The listing builds one solid part. Answer for the finished solid, in the listing's coordinates (mm). Face numbers are marked on the shaded views. Coordinates: 2 decimals unless noted, no trailing zeros. Write each loop counter-clockwise with the first axis right and the second up, starting at its lowest first coordinate (ties: lowest second). Pieces come first, ordered by that corner, then holes. Notation, with made-up numbers: M -10,-25 L 23,-25 A19 cw 23,-21 Z; hole C 87,36.25 d2. An arc over 180 degrees is marked long. Answer as CSV lines item,"result".
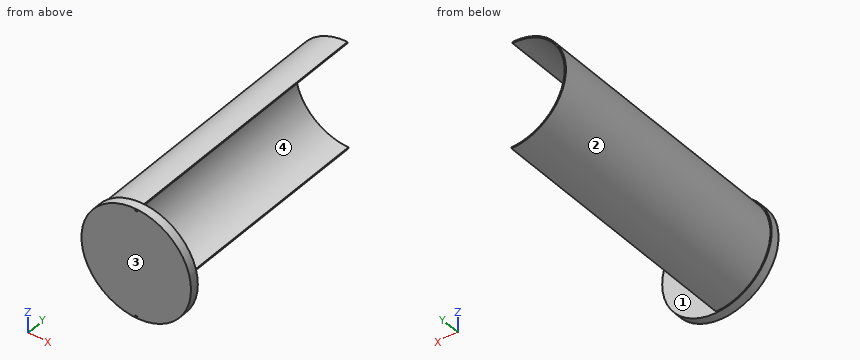
```python
from build123d import *

# Parameters (mm, degrees)
SKETCH1_R           = 62.5
BOSS_EXTRUDE2_DEPTH = 10
EXTRUDE_THIN1_DEPTH = 300
SKETCH8_W           = 3.337239336
SKETCH8_H           = 0.481982953
CUT_EXTRUDE1_DEPTH  = 311


with BuildPart() as part:
    # Sketch1 → Boss-Extrude2 (new body)
    with BuildSketch(Plane(origin=(0, 0, 0), x_dir=(1, 0, 0), z_dir=(0, 1, 0))):
        Circle(SKETCH1_R)
    extrude(amount=BOSS_EXTRUDE2_DEPTH)

    # Sketch4 → Extrude-Thin1 (add)
    with BuildSketch(Plane(origin=(0, 10, 0), x_dir=(1, 0, 0), z_dir=(0, 1, 0))):
        with BuildLine():
            ThreePointArc((0.99996418, 59.491596647), (-59.497899125, 0.499999744), (0, -59.5))
            Line((0, -59.5), (0, -61))
            ThreePointArc((0, -61), (-60.997846161, 0.51260478), (1.025173361, 60.991384798))
            Line((1.025173361, 60.991384798), (0.99996418, 59.491596647))
        make_face()
    extrude(amount=EXTRUDE_THIN1_DEPTH)

    # Sketch8 → Cut-Extrude1 (cut, through all)
    with BuildSketch(Plane(origin=(0, 310, 0), x_dir=(1, 0, 0), z_dir=(0, 1, 0))):
        with Locations((0.042875515, -60.380737202)):
            Rectangle(SKETCH8_W, SKETCH8_H)
    cut_extrude1 = extrude(amount=-CUT_EXTRUDE1_DEPTH, mode=Mode.SUBTRACT)

    # Mirror1: Cut-Extrude1 across plane
    add(cut_extrude1.mirror(Plane.XY), mode=Mode.SUBTRACT)


solid = part.part
```
Q1. Find section A-A (z = 0). Give the vertices of the cut face in (x, y), and give its area (3 significant figures).
Output:
outline,"M -62.5,0 L 62.5,0 L 62.5,10 L -59.5,10 L -59.5,310 L -61,310 L -61,10 L -62.5,10 Z"
area,"1,700 mm2"
Q2. The mould has two halves that part along Z. Classify the marked faces 1, 2, 3 and 4: pulls with the +Z half, pulls with the -Z half, needs draft (parallel to the pull), parting line crosses it, or undercut.
Output:
face 1,"undercut"
face 2,"parting line crosses it"
face 3,"needs draft"
face 4,"undercut"
Q3. Flat-ended cylindrical pins translate along their axes: pin 1 Ø4 at (x, z) = (9, -16) entering from +Y; pin 2 Ø1 at (x, y) = (-0.5, 118.5) entering from -Z; pin 3 Ø10 at (y, z) = (156, -5.5) entering from +X; pin 4 Ø1 at (x, z) = (-22, -33) entering from -Y. Find the tip coordinate at first contact, or state that the pin passes through.
Output:
pin 1,"y = 10"
pin 2,"z = -61"
pin 3,"x = -58.57"
pin 4,"y = 0"
Q4. Find section B-B (x = -19). Give the vertices of the cut face in (y, z), and give its area (3 significant figures).
Output:
outline,"M 0,-59.54 L 10,-59.54 L 10,-57.97 L 310,-57.97 L 310,-56.38 L 10,-56.38 L 10,56.38 L 310,56.38 L 310,57.97 L 10,57.97 L 10,59.54 L 0,59.54 Z"
area,"2,140 mm2"
Q5. Find section D-D (z = 16.5). Give the vertices of the cut face in (x, y), and give its area (3 significant figures).
Output:
outline,"M -60.28,0 L 60.28,0 L 60.28,10 L -57.17,10 L -57.17,310 L -58.73,310 L -58.73,10 L -60.28,10 Z"
area,"1,670 mm2"
Q6. Straight lines are drawn through the part: line 1 (Y direction, x = 56.5, z = 24.5); line 2 (X direction, y = 98, z = 2.5); line 3 (Z direction, x = -8, y = 263.5). For each, find the intervals that lie inside material, in ascending order.
Output:
line 1,"0 to 10"
line 2,"-60.95 to -59.45"
line 3,"-60.47 to -58.96, 58.96 to 60.47"
Q7. Find section C-C (y = 201.5). Give the vertices of the cut face in (x, z), and give its area (3 significant figures).
Output:
outline,"M -1.63,-60.62 L -1.63,-60.14 L 1.01,-60.14 L 1,-59.49 A59.5 cw long 0,59.5 L 0,60.14 L -1.63,60.14 L -1.63,60.62 L 0,60.62 L 0,61 A61 ccw long 1.03,-60.99 L 1.02,-60.62 Z"
area,"283 mm2"
